Can you work these out from the model? Positions are in its coordinate system, mm. Give positions to 0.01 mm unless a question says otherwise; leave off trailing zeros. Order: outer loops, then holes, each group sorted by start corner. A loop starts at its lowest first (then second) coordinate and runs counter-clockwise, first axis right, second up. Notation, with made-up numbers: (42.5, 27) -> (80.5, 27) arc R14 cw to (80.5, 45) -> close; hole circle Ø1 at (41.25, 88.5). An arc over 180 degrees is marked (long way). Answer as a JSON object with one key per item and string values.
```python
from build123d import *

# Parameters (mm, degrees)
F0_R     = 2.75
F0_R_2   = 9
F0_R_3   = 5.05
F1_DEPTH = 4


with BuildPart() as f1:
    # F0 (on Right) → F1 (new body)
    with BuildSketch(Plane.YZ):
        with BuildLine():
            Line((-8, -54), (8, -54))
            ThreePointArc((8, -54), (11.535534, -52.535534), (13, -49))
            Line((13, -49), (13, 49))
            ThreePointArc((13, 49), (11.535534, 52.535534), (8, 54))
            Line((8, 54), (-8, 54))
            ThreePointArc((-8, 54), (-11.535534, 52.535534), (-13, 49))
            Line((-13, 49), (-13, -49))
            ThreePointArc((-13, -49), (-11.535534, -52.535534), (-8, -54))
        make_face()
        with Locations((0, -49)):
            Circle(F0_R, mode=Mode.SUBTRACT)
        with Locations((0, -31)):
            Circle(F0_R_2, mode=Mode.SUBTRACT)
        with Locations((0, 9)):
            Circle(F0_R_2, mode=Mode.SUBTRACT)
        with Locations((0, 27)):
            Circle(F0_R, mode=Mode.SUBTRACT)
        with Locations((0, 44)):
            Circle(F0_R_3, mode=Mode.SUBTRACT)
    extrude(amount=F1_DEPTH)


solid = f1.part
```
1. If we section it at C-C on x = 1.45: Please give me the cut outline in (y, z), then the cut area to 3 significant figures.
Worked answers:
{"outline": "(-13, -49) arc R5 ccw to (-8, -54) -> (8, -54) arc R5 ccw to (13, -49) -> (13, 49) arc R5 ccw to (8, 54) -> (-8, 54) arc R5 ccw to (-13, 49) -> close; hole circle Ø18 at (0, -31); hole circle Ø18 at (0, 9); hole circle Ø10.1 at (0, 44); hole circle Ø5.5 at (0, -49); hole circle Ø5.5 at (0, 27)", "area": "2,150 mm²"}
2. Please list where these lines run through material, in increasing order: L1, parallel to Z at x = 2.15, y = 0; L2, parallel to Z at x = 1.4, y = 5.75; L3, parallel to Z at x = 0.95, y = 4.
Worked answers:
{"L1": "-54 to -51.75, -46.25 to -40, -22 to 0, 18 to 24.25, 29.75 to 38.95, 49.05 to 54", "L2": "-54 to -37.92, -24.08 to 2.08, 15.92 to 54", "L3": "-54 to -39.06, -22.94 to 0.94, 17.06 to 40.92, 47.08 to 54"}
3. If we section it at B-B on z = 44: Please give me the cut outline in (x, y), then the cut area to 3 significant figures.
Worked answers:
{"outline": "(0, -13) -> (4, -13) -> (4, -5.05) -> (0, -5.05) -> close; (0, 5.05) -> (4, 5.05) -> (4, 13) -> (0, 13) -> close", "area": "63.6 mm²"}
4. If we mould it in two halves opening along Y, with no side actions, what happens to faces 1 (the face through (2, -12, -52)), 2 (the face through (2, 0, 54)), 3 (the face through (1.972, -1.172, -22.077))? For each: +Y half, -Y half, draft (parallel to the pull), parting line (faces both ways), or undercut.
Worked answers:
{"face 1": "-Y half", "face 2": "draft", "face 3": "undercut"}
5. If we section it at A-A on y = 0: Please give me the cut outline in (x, z), then the cut area to 3 significant figures.
Worked answers:
{"outline": "(0, -54) -> (4, -54) -> (4, -51.75) -> (0, -51.75) -> close; (0, -46.25) -> (4, -46.25) -> (4, -40) -> (0, -40) -> close; (0, -22) -> (4, -22) -> (4, 0) -> (0, 0) -> close; (0, 18) -> (4, 18) -> (4, 24.25) -> (0, 24.25) -> close; (0, 29.75) -> (4, 29.75) -> (4, 38.95) -> (0, 38.95) -> close; (0, 49.05) -> (4, 49.05) -> (4, 54) -> (0, 54) -> close", "area": "204 mm²"}
6. If we section it at D-D on z = 9: Please give me the cut outline in (x, y).
Worked answers:
{"outline": "(0, -13) -> (4, -13) -> (4, -9) -> (0, -9) -> close; (0, 9) -> (4, 9) -> (4, 13) -> (0, 13) -> close"}
